Design review of the part shown in the three views and the two pictorial views. Dimensions are in mm from the part's minimum x, y and z. Round coordinates to 2 decimals unless told otherwise and drop trailing zeros. Write each loop counter-clockwise with the first axis right and the second up, starting at its lowest first coordinate (ties: lowest second). Pieces come first, ordered by that corner, then holes. Notation, with made-up numbers: (46, 60) -> (104, 60) arc R29 cw to (104, 91) -> close; hole circle Ø3 at (86, -10). An arc over 180 degrees is marked (long way). Answer as a JSON object with one key per item and string values. Group by question number.
1) We need section A-A, the plane x = 12.7. Write out the cut boundary in (y, z).
2) To check wall thickness, follow probe 1 along X at (y, z) = (12.7, 1.1); probe 2 along Y at (x, z) = (19.5, 1.6). State the ranges of each line that lie inside material, in increasing order. Write a range as [from, to].
3) We need section C-C, the plane z = 3.2. Count the separate pieces of the cut face and the enclosed holes in it, then the cut area to 3 significant figures.
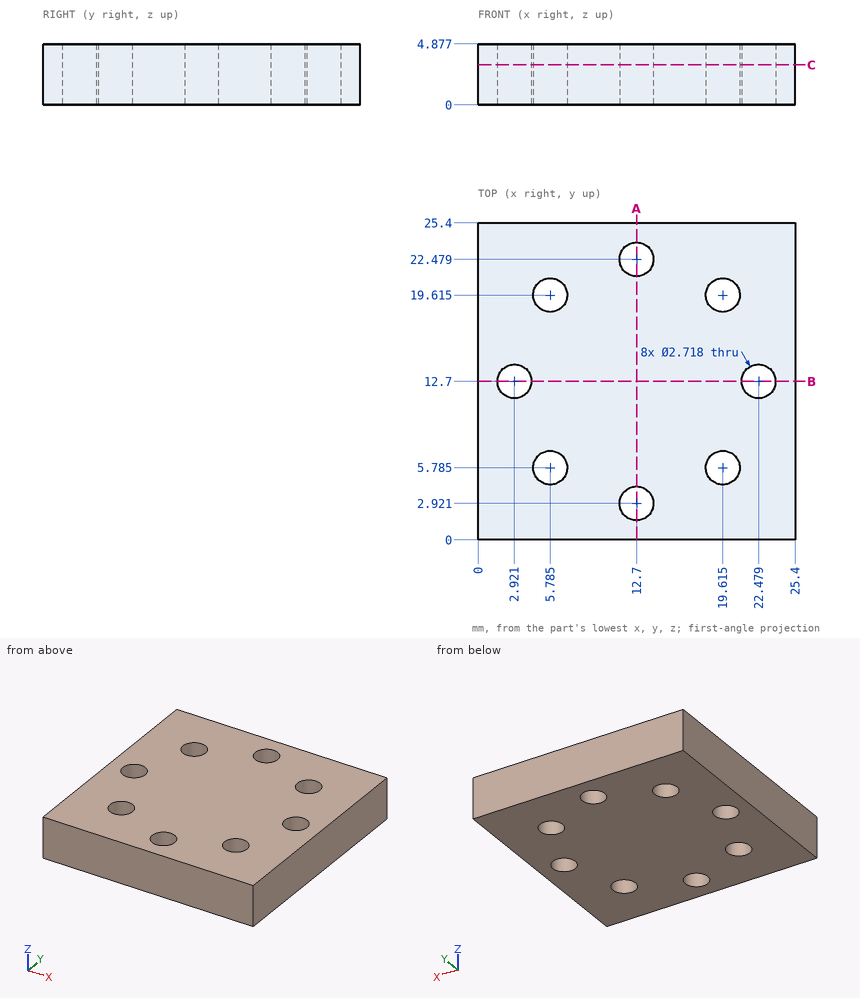
Here are the results:
{
 "1": {"outline": "(0, 0) -> (1.56, 0) -> (1.56, 4.88) -> (0, 4.88) -> close; (4.28, 0) -> (21.12, 0) -> (21.12, 4.88) -> (4.28, 4.88) -> close; (23.84, 0) -> (25.4, 0) -> (25.4, 4.88) -> (23.84, 4.88) -> close"},
 "2": {"probe 1": "x = [0, 1.56], [4.28, 21.12], [23.84, 25.4]", "probe 2": "y = [0, 4.43], [7.14, 18.26], [20.97, 25.4]"},
 "3": {"separate pieces": "1", "enclosed holes": "8", "area": "599 mm^2"}
}
